from build123d import *

# Parameters (mm, degrees)
EXTRUDE_1_DEPTH          = 24
CUT_EXTRUDE_1_DEPTH      = 24
CUT_EXTRUDE_1_DEPTH_BACK = 24
SKETCH_2_R               = 2
CUT_EXTRUDE_2_DEPTH      = 24
CUT_EXTRUDE_2_DEPTH_BACK = 24
SKETCH_3_R               = 2


with BuildPart() as part:
    # Эскиз1 → Бобышка-Вытянуть1 (new body)
    with BuildSketch(Plane(origin=(0, 0, 0), x_dir=(0, 0, -1), z_dir=(1, 0, 0))):
        Polygon((0, 0), (-26, 0), (-26, 2), (-2, 2), (-2, 26), (0, 26), align=None)
    extrude(amount=EXTRUDE_1_DEPTH)

    # Эскиз2 → Вырез-Вытянуть1 (cut, two sides: drawn at the far end of the back side and taken through both)
    with BuildSketch(Plane.XY.offset(-CUT_EXTRUDE_1_DEPTH_BACK)):
        with Locations(Location((12, 14, 0), (0, 0, 90))):
            Circle(SKETCH_2_R)
        with Locations(Location((4, 14, 0), (0, 0, 90))):
            Circle(SKETCH_2_R)
        with Locations(Location((20, 14, 0), (0, 0, 90))):
            Circle(SKETCH_2_R)
        with Locations(Location((12, 22, 0), (0, 0, 90))):
            Circle(SKETCH_2_R)
        with Locations(Location((4, 22, 0), (0, 0, 90))):
            Circle(SKETCH_2_R)
        with Locations(Location((20, 22, 0), (0, 0, 90))):
            Circle(SKETCH_2_R)
        with Locations(Location((12, 6, 0), (0, 0, 90))):
            Circle(SKETCH_2_R)
        with Locations(Location((4, 6, 0), (0, 0, 90))):
            Circle(SKETCH_2_R)
        with Locations(Location((20, 6, 0), (0, 0, 90))):
            Circle(SKETCH_2_R)
        with BuildLine():
            Line((0, 26), (0, 25))
            ThreePointArc((0, 25), (0.292893219, 25.707106781), (1, 26))
            Line((1, 26), (0, 26))
        make_face()
        with BuildLine():
            Line((24, 26), (23, 26))
            ThreePointArc((23, 26), (23.707106781, 25.707106781), (24, 25))
            Line((24, 25), (24, 26))
        make_face()
    extrude(amount=CUT_EXTRUDE_1_DEPTH + CUT_EXTRUDE_1_DEPTH_BACK, mode=Mode.SUBTRACT)

    # Эскиз3 → Вырез-Вытянуть2 (cut, two sides: drawn at the far end of the back side and taken through both)
    with BuildSketch(Plane(origin=(0, 0, 0), x_dir=(1, 0, 0), z_dir=(0, 1, 0)).offset(-CUT_EXTRUDE_2_DEPTH_BACK)):
        with Locations(Location((12, -14, 0), (0, 0, 90))):
            Circle(SKETCH_3_R)
        with Locations(Location((4, -14, 0), (0, 0, 90))):
            Circle(SKETCH_3_R)
        with Locations(Location((20, -14, 0), (0, 0, 90))):
            Circle(SKETCH_3_R)
        with Locations(Location((12, -6, 0), (0, 0, 90))):
            Circle(SKETCH_3_R)
        with Locations(Location((4, -6, 0), (0, 0, 90))):
            Circle(SKETCH_3_R)
        with Locations(Location((20, -6, 0), (0, 0, 90))):
            Circle(SKETCH_3_R)
        with Locations(Location((12, -22, 0), (0, 0, 90))):
            Circle(SKETCH_3_R)
        with Locations(Location((4, -22, 0), (0, 0, 90))):
            Circle(SKETCH_3_R)
        with Locations(Location((20, -22, 0), (0, 0, 90))):
            Circle(SKETCH_3_R)
        with BuildLine():
            Line((0, -25), (0, -26))
            Line((0, -26), (1, -26))
            ThreePointArc((1, -26), (0.292893219, -25.707106781), (0, -25))
        make_face()
        with BuildLine():
            Line((24, -26), (23, -26))
            ThreePointArc((23, -26), (23.707106781, -25.707106781), (24, -25))
            Line((24, -25), (24, -26))
        make_face()
    extrude(amount=CUT_EXTRUDE_2_DEPTH + CUT_EXTRUDE_2_DEPTH_BACK, mode=Mode.SUBTRACT)


solid = part.part
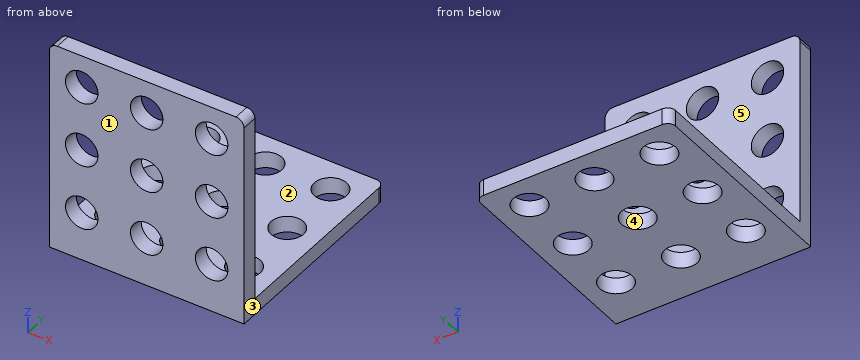
Design review of the part built by this model. Coordinates are the model's own, in mm. Face numbers are marked on the shaded views. A direction names the side the tool comes from. Coordinates: 2 decimals unless noted, no trailing zeros. Loops run counter-clockwise (first coordinate to the right, second up) from the corner with the lowest first, then second, coordinate; pieces in that order, holes last. Notation, with made-up numbers: (87, 58) -> (139, 58) arc R7 ccw to (139, 64) -> close; hole circle Ø11 at (66, 80.5). An arc over 180 degrees is marked (long way). Use a Markdown table: item, result. Add a question column.
Item 1: We need section D-D, the plane x = 8. Write out the cut boundary in (y, z), and give its area (3 significant figures).
Item 2: Wall thickness on L1, parallel to X at y = 0.55, z = 14; L2, parallel to Y at x = 18.75, z = 1.75; L3, parallel to Z at x = 23, y = 18.5: over which ranges is each line inside the solid? List them lowest first. Write a range as from..to.
Item 3: Machinability: for the marked faces 1 and 2, which of the approach directions +Z, -Z, +X, -X, +Y, -Y give a long, thin tool a straight path to every point of the face, cutting with its end or side? Answer none if there is none.
Item 4: The part is to be moulded in two halves that separate along X. For the marked faces 3, 4 and 5, say which applies: +X half, -X half, draft (parallel to the pull), parting line (faces both ways), or undercut.
Item 5: We need section B-B, the plane y = 22. Write out the cut boundary in (x, z), and give its area (3 significant figures).
Item 6: We need section A-A, the plane z = 1.5. Count the separate pieces of the cut face and the enclosed holes in it, and give its area (3 significant figures).
Item 7: Clearance check with flat-ended pins moving along their axes: P1, Ø1.5, axis at x = 18.5, y = 13.5, coming from the +Z side; P2, Ø4.5, axis at x = 20, y = 14, coming from the -Z side; P3, Ø2, axis at x = 9, z = 9, coming from the +Y side. State where each tip first meets the part, or that it passes through.
Item 8: We need section C-C, the plane z = 13.75. Write out the cut boundary in (x, y).
Numbers:
| question | item | result |
|---|---|---|
| 1 | outline | (0, 0) -> (26, 0) -> (26, 2) -> (2, 2) -> (2, 26) -> (0, 26) -> close |
| 1 | area | 100 mm^2 |
| 2 | L1 | x = 0..2, 6..10, 14..18, 22..24 |
| 2 | L2 | y = 0..4.44, 7.56..12.44, 15.56..20.44, 23.56..26 |
| 2 | L3 | z = 0..2 |
| 3 | face 1 | +Z, -Z, +X, -X, -Y |
| 3 | face 2 | +Z, +X, -X, +Y |
| 4 | face 3 | +X half |
| 4 | face 4 | undercut |
| 4 | face 5 | draft |
| 5 | outline | (0, 0) -> (2, 0) -> (2, 2) -> (0, 2) -> close; (6, 0) -> (10, 0) -> (10, 2) -> (6, 2) -> close; (14, 0) -> (18, 0) -> (18, 2) -> (14, 2) -> close; (22, 0) -> (24, 0) -> (24, 2) -> (22, 2) -> close |
| 5 | area | 24.0 mm^2 |
| 6 | separate pieces | 1 |
| 6 | enclosed holes | 9 |
| 6 | area | 510 mm^2 |
| 7 | P1 | stops at z = 2 |
| 7 | P2 | stops at z = 0 |
| 7 | P3 | stops at y = 2 |
| 8 | outline | (0, 0) -> (2.02, 0) -> (2.02, 2) -> (0, 2) -> close; (5.98, 0) -> (10.02, 0) -> (10.02, 2) -> (5.98, 2) -> close; (13.98, 0) -> (18.02, 0) -> (18.02, 2) -> (13.98, 2) -> close; (21.98, 0) -> (24, 0) -> (24, 2) -> (21.98, 2) -> close |
